from build123d import *

# Parameters (mm, degrees)
SKETCH1_W          = 40
SKETCH1_H          = 43.18
BASE_DEPTH         = 2.4638
SKETCH2_W          = 12.7
SKETCH2_H          = 2.4638
BOTTOM_TABS_DEPTH  = 5.334
MOUNT_POINTS_DEPTH = 59.911651737
SKETCH6_R          = 4.245
CUT_EXTRUDE2_DEPTH = 66.894365141


with BuildPart() as part:
    # Sketch1 → Base (new body)
    with BuildSketch(Plane.XY):
        with Locations((20, 21.59)):
            Rectangle(SKETCH1_W, SKETCH1_H)
    extrude(amount=BASE_DEPTH)

    # Sketch2 → Bottom Tabs (add)
    with BuildSketch(Plane.XZ):
        with Locations((6.35, 1.2319)):
            Rectangle(SKETCH2_W, SKETCH2_H)
        with Locations((33.65, 1.2319)):
            Rectangle(SKETCH2_W, SKETCH2_H)
    extrude(amount=BOTTOM_TABS_DEPTH)

    # Sketch4 → Mount Points (cut, through all)
    with BuildSketch(Plane.XY.offset(2.4638)):
        with BuildLine():
            Line((31.481992586, 29.154809731), (32.871526584, 30.54434373))
            Line((32.871526584, 30.54434373), (29.061376273, 34.354494041))
            Line((29.061376273, 34.354494041), (27.693229207, 32.986346975))
            ThreePointArc((27.693229207, 32.986346975), (10.22286074, 11.922009108), (31.481992586, 29.154809731))
        make_face()
    extrude(amount=-MOUNT_POINTS_DEPTH, mode=Mode.SUBTRACT)

    # Sketch6 → Cut-Extrude2 (cut, through all)
    with BuildSketch(Plane(origin=(18.246403628, 22.293576812, 55.7276), x_dir=(1, 0, 0), z_dir=(0, 0, 1))):
        with Locations((15.813596372, 23.649057543)):
            Circle(SKETCH6_R)
    extrude(amount=-CUT_EXTRUDE2_DEPTH, mode=Mode.SUBTRACT)


solid = part.part
Model file for the job. Use its own axes, mm. A direction names the side the tool comes from. Give positions to 0.01 mm unless a question says otherwise; leave off trailing zeros. Order: outer loops, then holes, each group sorted by start corner. A loop starts at its lowest first (then second) coordinate and runs counter-clockwise, first axis right, second up. Notation, with made-up numbers: (-21.5, 62.5) - (-1.5, 62.5) arc R8 ccw to (-1.5, 67.5) - close; hole circle Ø11 at (73, 20). An arc over 180 degrees is marked (long way). Write item = value, one per line. Start each with the question number.
1. Two-plate mould, pull along X, no slides. Class faces 1 (the flat face through (15, 43.18, 1)), 2 (the flat face through (0, 19, 1)), 3 (the cylindrical face through (9.833, 12.333, 1.249)), 4 (the flat face through (28.387, 33.68, 1.249)): pulls with the +X half, pulls with the -X half, needs draft (parallel to the pull), parting line crosses it, or undercut.
2. Cut at B-B, the plane y = 21.59. List the corners of the cut face in (x, z), and give its area (3 significant figures).
3. Probe line 1 along Y through (x, z) = (20, 0.85); line 2 along X through (y, z) = (21.59, 1.15); line 3 along X through (y, z) = (-0.5, 1.8). List the from-to ranges inside material, lowest first.
4. Which spindle directions (+Z, -Z, +X, -X, +Y, -Y) get a long thin tool onto all of the face, cutting with end or side? Do faces 5 (the cylindrical face through (34, 41.7, 1.2)), 6 (the flat face through (32.17, 29.84, 1.25)), 7 (the flat face through (20, 0, 1)). Say none if no direction does.
5. Cut at A-A, the plane x = 20. List the corners of the cut face in (y, z), and give its area (3 significant figures).
Taken from the geometry:
q1.face_1 = needs draft
q1.face_2 = pulls with the -X half
q1.face_3 = undercut
q1.face_4 = undercut
q2.outline = (0, 0) - (6.25, 0) - (6.25, 2.46) - (0, 2.46) - close; (33.75, 0) - (40, 0) - (40, 2.46) - (33.75, 2.46) - close
q2.area = 30.8 mm²
q3.line_1 = 0 to 7.84, 35.34 to 43.18
q3.line_2 = 0 to 6.25, 33.75 to 40
q3.line_3 = 0 to 12.7, 27.3 to 40
q4.face_5 = +Z, -Z, +Y
q4.face_6 = +Z, -Z
q4.face_7 = +Z, -Z, -Y
q5.outline = (0, 0) - (7.84, 0) - (7.84, 2.46) - (0, 2.46) - close; (35.34, 0) - (43.18, 0) - (43.18, 2.46) - (35.34, 2.46) - close
q5.area = 38.6 mm²
